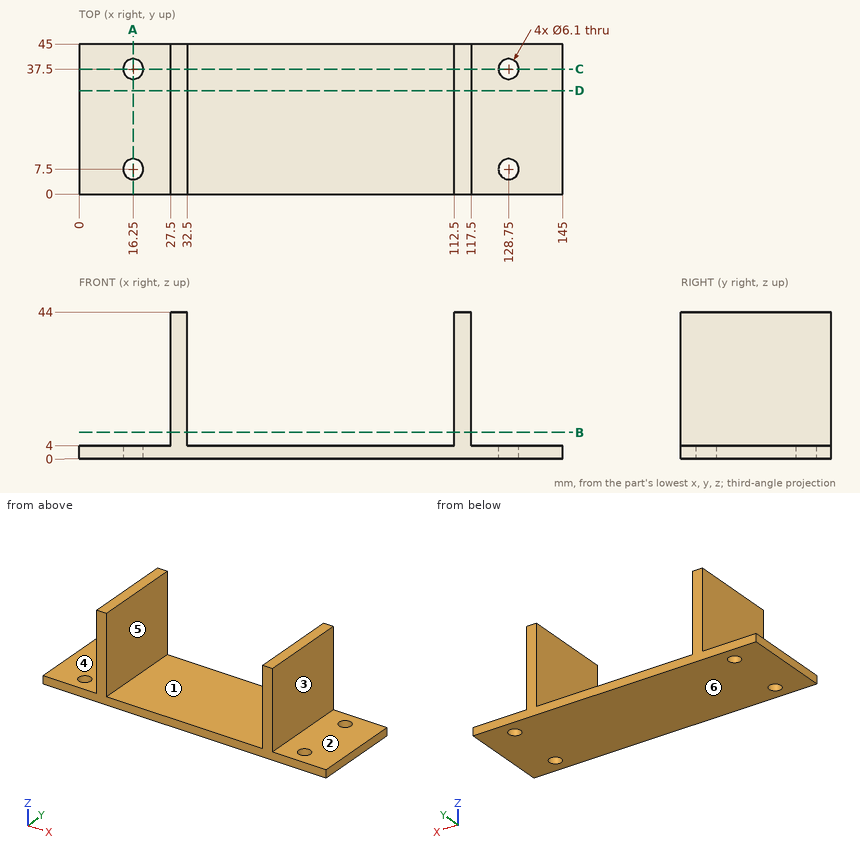
The drawing under review shows one solid part. Ordinate dimensions are in mm from its lowest x, y, z. A direction names the side the tool comes from. Round coordinates to 2 decimals unless told otherwise and drop trailing zeros. Loops run counter-clockwise (first coordinate to the right, second up) from the corner with the lowest first, then second, coordinate; pieces in that order, holes last. Notation, with made-up numbers: (21, 13) - (46, 13) arc R26 cw to (46, 52) - close; hole circle Ø10 at (30.25, 6). An arc over 180 degrees is marked (long way). Use a Markdown table: item, result. Add a question column.
Q1. Add section B-B (z = 8). State the section outline as (x, y) points, plus the area to 3 significant figures.
Q2. The part is to be moulded in two halves that separate along X. For the marked faces 1, 2 and 3, say which applies: pulls with the +X half, pulls with the -X half, needs draft (parallel to the pull), parting line crosses it, or undercut.
Q3. Add section D-D (y = 31). State the section outline as (x, z) points.
Q4. Add section A-A (x = 16.25). State the section outline as (y, z) points, plus the area to 3 significant figures.
Q5. Add section C-C (y = 37.5). State the section outline as (x, z) points.
Q6. Insertion check: pin 1 Ø10 at (x, y) = (128.75, 37.5) entering from +Z; pin 2 Ø6 at (y, z) = (14.5, 13.5) entering from +X; pin 3 Ø5 at (y, z) = (27, 10.5) entering from -X; pin 4 Ø6 at (x, y) = (104, 14.5) entering from -Z. Each pin has a flat end and moves straight along its axis. Give the tip position at first contact, or say it passes through.
Q7. For probe 1 along Y at (x, z) = (128.75, 2.7); probe 2 along X at (y, z) = (41.5, 9.5); probe 3 along X at (y, z) = (37, 1), list the stretches that pass through material, from the lowest coordinate up.
Q8. Machinability: for the marked faces 4, 5 and 6, which of the approach directions +Z, -Z, +X, -X, +Y, -Y give a long, thin tool a straight path to every point of the face, cutting with its end or side? Answer none if there is none.
Worked answers:
| question | item | result |
|---|---|---|
| 1 | outline | (27.5, 0) - (32.5, 0) - (32.5, 45) - (27.5, 45) - close; (112.5, 0) - (117.5, 0) - (117.5, 45) - (112.5, 45) - close |
| 1 | area | 450 mm² |
| 2 | face 1 | undercut |
| 2 | face 2 | needs draft |
| 2 | face 3 | pulls with the +X half |
| 3 | outline | (0, 0) - (145, 0) - (145, 4) - (117.5, 4) - (117.5, 44) - (112.5, 44) - (112.5, 4) - (32.5, 4) - (32.5, 44) - (27.5, 44) - (27.5, 4) - (0, 4) - close |
| 4 | outline | (0, 0) - (4.45, 0) - (4.45, 4) - (0, 4) - close; (10.55, 0) - (34.45, 0) - (34.45, 4) - (10.55, 4) - close; (40.55, 0) - (45, 0) - (45, 4) - (40.55, 4) - close |
| 4 | area | 131 mm² |
| 5 | outline | (0, 0) - (13.2, 0) - (13.2, 4) - (0, 4) - close; (19.3, 0) - (125.7, 0) - (125.7, 4) - (117.5, 4) - (117.5, 44) - (112.5, 44) - (112.5, 4) - (32.5, 4) - (32.5, 44) - (27.5, 44) - (27.5, 4) - (19.3, 4) - close; (131.8, 0) - (145, 0) - (145, 4) - (131.8, 4) - close |
| 6 | pin 1 | z = 4 |
| 6 | pin 2 | x = 117.5 |
| 6 | pin 3 | x = 27.5 |
| 6 | pin 4 | z = 0 |
| 7 | probe 1 | 0 to 4.45, 10.55 to 34.45, 40.55 to 45 |
| 7 | probe 2 | 27.5 to 32.5, 112.5 to 117.5 |
| 7 | probe 3 | 0 to 13.24, 19.26 to 125.74, 131.76 to 145 |
| 8 | face 4 | +Z, -X, +Y, -Y |
| 8 | face 5 | +Z, +Y, -Y |
| 8 | face 6 | -Z, +X, -X, +Y, -Y |
